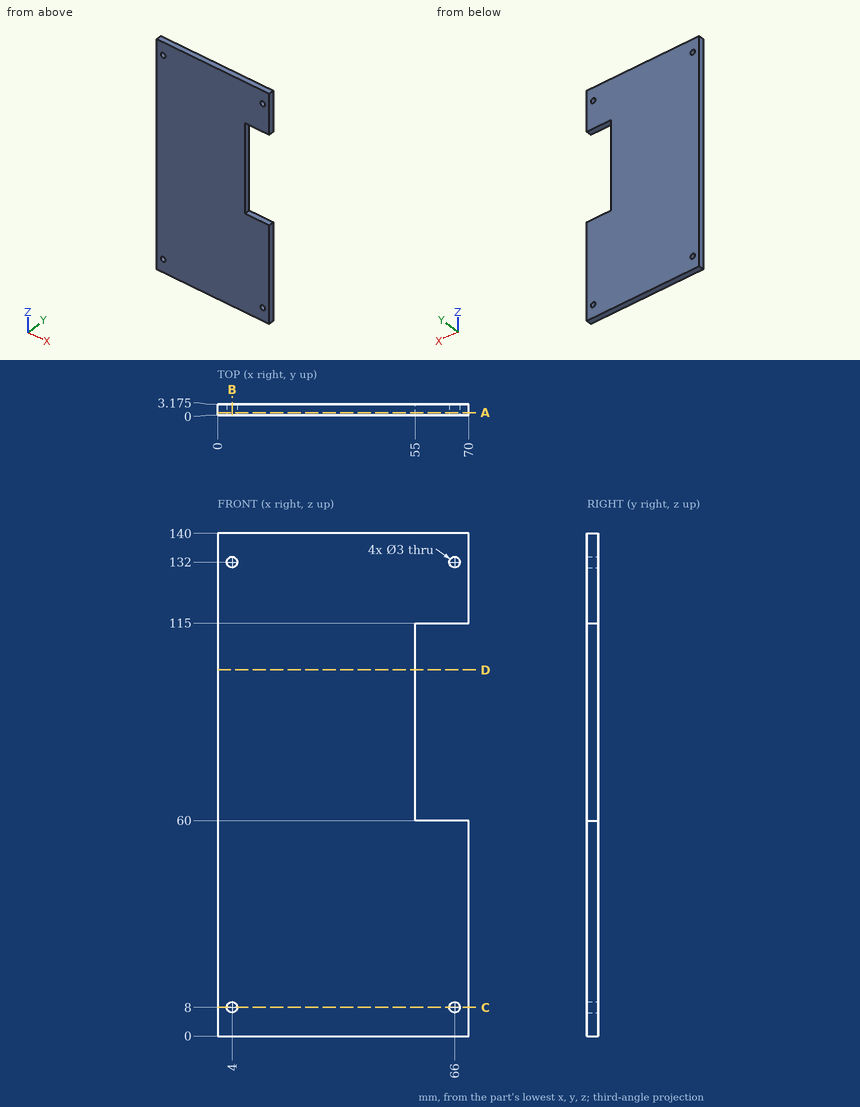
Could you check a few things on this drawing? It's one solid part, dimensions in mm from its lowest x, y, z. Coordinates: 2 decimals unless noted, no trailing zeros. Order: outer loops, then holes, each group sorted by start corner. A loop starts at its lowest first (then second) coordinate and runs counter-clockwise, first axis right, second up. Notation, with made-up numbers: (85, 86) -> (127, 86) arc R24 ccw to (127, 118) -> close; hole circle Ø7 at (63.5, 8). An arc over 180 degrees is marked (long way). One line per item, written item: value. Start each with the question number.
1) If I drill on L1, parallel to X at y = 1.4, z = 132; L2, parallel to Z at x = 66, y = 1.6; L3, parallel to Z at x = 63, y = 2.2, over which ranges is the centre line in solid material (lowest first)? Write a range as [from, to].
2) Imagine slicing it at B-B on x = 4. List the corners of the cut face in (y, z) for me (3 decimals).
3) Imagine slicing it at A-A on y = 0.8. List the corners of the cut face in (x, z) for me, plus the area to 3 significant figures.
4) Imagine slicing it at D-D on z = 102. List the corners of the cut face in (x, y) for me (3 decimals).
5) Imagine slicing it at C-C on z = 8. List the corners of the cut face in (x, y) for me (3 decimals), plus the area to 3 significant figures.
Answer list:
1. L1: x = [0, 2.5], [5.5, 64.5], [67.5, 70]
1. L2: z = [0, 6.5], [9.5, 60], [115, 130.5], [133.5, 140]
1. L3: z = [0, 60], [115, 140]
2. outline: (0, 0) -> (3.175, 0) -> (3.175, 6.5) -> (0, 6.5) -> close; (0, 9.5) -> (3.175, 9.5) -> (3.175, 130.5) -> (0, 130.5) -> close; (0, 133.5) -> (3.175, 133.5) -> (3.175, 140) -> (0, 140) -> close
3. outline: (0, 0) -> (70, 0) -> (70, 60) -> (55, 60) -> (55, 115) -> (70, 115) -> (70, 140) -> (0, 140) -> close; hole circle Ø3 at (4, 8); hole circle Ø3 at (4, 132); hole circle Ø3 at (66, 8); hole circle Ø3 at (66, 132)
3. area: 8,950 mm2
4. outline: (0, 0) -> (55, 0) -> (55, 3.175) -> (0, 3.175) -> close
5. outline: (0, 0) -> (2.5, 0) -> (2.5, 3.175) -> (0, 3.175) -> close; (5.5, 0) -> (64.5, 0) -> (64.5, 3.175) -> (5.5, 3.175) -> close; (67.5, 0) -> (70, 0) -> (70, 3.175) -> (67.5, 3.175) -> close
5. area: 203 mm2
